```python
from build123d import *

# Parameters (mm, degrees)
SKETCH1_R                         = 8
BLADE_HOLDER_EXTRUDE_DEPTH        = 1
SKETCH2_R                         = 7
BLADE_HOLDER_EXTRUDE_2_DEPTH      = 2
SKETCH3_R                         = 6
BLADE_HOLDER_EXTRUDE_3_DEPTH      = 4
SKETCH4_R                         = 1
HOLE_FOR_SCREW_BLADE_HOLDER_DEPTH = 24
BLADE_HOLDER_FILLET_1_R           = 1
BLADE_HOLDER_FILLET_2_R           = 2.5


# Some blends are built 0.0001 mm under size
with BuildPart() as part:
    # Sketch1 → Blade Holder Extrude (new body)
    with BuildSketch(Plane(origin=(0, 0, 0), x_dir=(1, 0, 0), z_dir=(0, 1, 0))):
        with Locations(Location((0, 0, 0), (0, 0, 270))):
            Circle(SKETCH1_R)
    extrude(amount=BLADE_HOLDER_EXTRUDE_DEPTH)

    # Sketch2 → Blade Holder Extrude 2 (add)
    with BuildSketch(Plane(origin=(0, 1, 0), x_dir=(1, 0, 0), z_dir=(0, 1, 0))):
        with Locations(Location((0, 0, 0), (0, 0, 270))):
            Circle(SKETCH2_R)
    extrude(amount=BLADE_HOLDER_EXTRUDE_2_DEPTH)

    # Sketch3 → Blade Holder Extrude 3 (add)
    with BuildSketch(Plane(origin=(0, 3, 0), x_dir=(1, 0, 0), z_dir=(0, 1, 0))):
        with Locations(Location((0, 0, 0), (0, 0, 270))):
            Circle(SKETCH3_R)
    extrude(amount=BLADE_HOLDER_EXTRUDE_3_DEPTH)

    # Sketch4 → Hole for Screw (Blade Holder) (cut)
    with BuildSketch(Plane(origin=(0, 7, 0), x_dir=(1, 0, 0), z_dir=(0, 1, 0))):
        with Locations(Location((0, 0, 0), (0, 0, 270))):
            Circle(SKETCH4_R)
    extrude(amount=-HOLE_FOR_SCREW_BLADE_HOLDER_DEPTH, mode=Mode.SUBTRACT)

    # Blade Holder Fillet 1
    blade_holder_fillet_1_edges = [part.edges().sort_by_distance(p)[0] for p in [
        (0, 1, -8),
    ]]
    fillet(blade_holder_fillet_1_edges, radius=BLADE_HOLDER_FILLET_1_R - 0.0001)  # a hair under: the kernel refuses the full size

    # Blade Holder Fillet 2
    # the kernel refuses this fillet: 2.5 mm, written as the material it takes off along each edge
    with BuildSketch(Plane(origin=(0, 3, 0), x_dir=(0, 0, 1), z_dir=(-1, 0, 0))) as blade_holder_fillet_2_piece_1:
        with BuildLine():
            CenterArc((4.5, -2), BLADE_HOLDER_FILLET_2_R, 0, 53.130102354)
            Line((6, 0), (7, 0))
            Line((7, 0), (7, -2))
        make_face()
    revolve(axis=Axis((0, 3, 0), (0, 1, 0)), mode=Mode.SUBTRACT)


solid = part.part
```
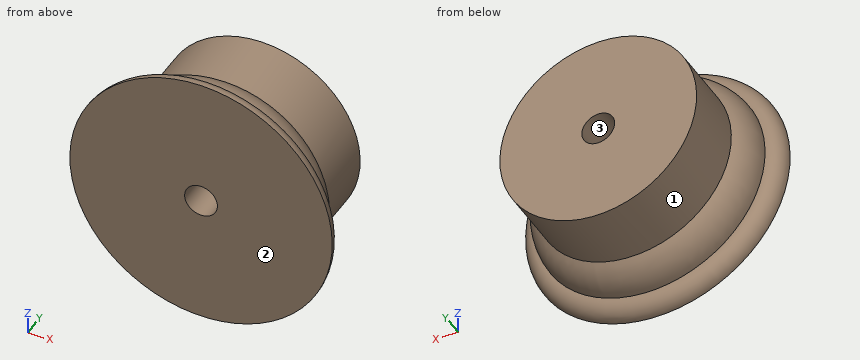
The listing builds one solid part. Answer for the finished solid, in the listing's coordinates (mm). Face numbers are marked on the shaded views. Give positions to 0.01 mm unless a question says otherwise; leave off trailing zeros. Write each loop counter-clockwise with the first axis right and the second up, starting at its lowest first coordinate (ties: lowest second). Pieces come first, ordered by that corner, then holes. Notation, with made-up numbers: (15, 1) -> (63, 1) arc R16 cw to (63, 29) -> close; hole circle Ø7 at (40, -17). An arc over 180 degrees is marked (long way). Use one line per item in the form item = value.
1) Each of these flat-tipped pins is pushed along its axis until it touches: P1, Ø2.5, axis at x = 0, z = 0, coming from the -Y side; P2, Ø3, axis at y = 2, z = -3, coming from the +X side; P3, Ø1.5, axis at x = -4.5, y = 2.5, coming from the +Z side. Where does it stop, or does it pass through?
Result:
P1 = 0
P2 = 7.4
P3 = 5.53
2) For a pull along Z with two mould halves and no side action, classify the marked faces 1, 2 and 3 as +Z half, -Z half, draft (parallel to the pull), parting line (faces both ways), or undercut.
Result:
face_1 = parting line
face_2 = draft
face_3 = undercut
3) Straight lines are drawn through the part: probe 1 along X at (y, z) = (5.25, 0); probe 2 along Y at (x, z) = (-6.5, -2); probe 3 along Z at (x, y) = (-4.5, 3.75). For each, find the intervals that lie inside material, in ascending order.
Result:
probe_1 = -6 to -1, 1 to 6
probe_2 = 0 to 1.98
probe_3 = -3.97 to 3.97
4) Section C-C on y = 3.5 is taken. Write down the section's boundary in (x, z), plus the area to 3 significant figures.
Result:
outline = circle Ø12 at (0, 0); hole circle Ø2 at (0, 0)
area = 110 mm²
